Source: CAD feature listing. Evaluate the final solid. Frame: model axes, mm. Face numbers are marked on the shaded views. Give positions to 0.01 mm unless a question says otherwise; leave off trailing zeros. Order: outer loops, then holes, each group sorted by start corner. A loop starts at its lowest first (then second) coordinate and runs counter-clockwise, first axis right, second up. Notation, with made-up numbers: (55.25, -18.5) - (96.25, -18.5) arc R13 cw to (96.25, 5.5) - close; hole circle Ø9 at (27.25, -9.5). An arc over 180 degrees is marked (long way). Write each question's results on one line, items separated by ' | '. Start each with the question number.
Item 1: Section A-A on x = -10.75. Output: boundary loops of the cut face in (y, z), and give its area (3 significant figures).
Item 2: Section B-B on y = 0. Output: boundary loops of the cut face in (x, z) (3 decimals), and give its area (3 significant figures).
Item 3: Section D-D on x = 10.75. Output: boundary loops of the cut face in (y, z) (3 decimals), and give its area (3 significant figures).
Item 4: Section C-C on z = 17.5. Output: boundary loops of the cut face in (x, y).
Item 5: Line query: line 1 along Y through (x, z) = (-10.75, 12.75); line 2 along X through (y, z) = (-2, 14); line 3 along X through (y, z) = (-0.5, 6.75). Output: solid intervals per line, ascending.
Item 6: Mould query, pull axis X, two halves, no side actions, for the marked faces 1, 2, 3 and 4. Classes: released by +X, released by -X, zero draft, split by the parting line, or undercut.
```python
from build123d import *

# Parameters (mm, degrees)
SKETCH_1_W                   = 40
SKETCH_1_H                   = 20
EXTRUDE_1_DEPTH              = 20
HOLE_WIZARD_M6_1_D           = 5
HOLE_WIZARD_M6_1_CSINK_D     = 6.05
HOLE_WIZARD_M6_1_CSINK_ANGLE = 90
SKETCH_3_R                   = 3
CUT_EXTRUDE_1_DEPTH          = 31


with BuildPart() as part:
    # 草图1 → 凸台-拉伸1 (new body)
    with BuildSketch(Plane.XY):
        Rectangle(SKETCH_1_W, SKETCH_1_H)
    extrude(amount=EXTRUDE_1_DEPTH)

    # M6 螺纹孔1 (through all)
    with Locations(Plane(origin=(10.75, 0, 0), x_dir=(-1, 0, 0), z_dir=(0, 0, -1))):
        with Locations((0, 0)):
            CounterSinkHole(HOLE_WIZARD_M6_1_D / 2, HOLE_WIZARD_M6_1_CSINK_D / 2, counter_sink_angle=HOLE_WIZARD_M6_1_CSINK_ANGLE)

    # 草图3 → 切除-拉伸1 (cut, through all)
    with BuildSketch(Plane.XY.offset(20)):
        with Locations((-10.75, 0)):
            Circle(SKETCH_3_R)
    extrude(amount=-CUT_EXTRUDE_1_DEPTH, mode=Mode.SUBTRACT)


solid = part.part
```
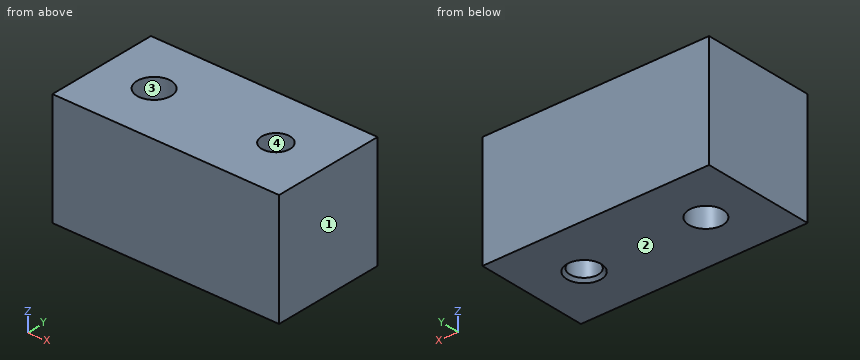
Evaluation:
1) outline: (-10, 0) - (-3, 0) - (-3, 20) - (-10, 20) - close; (3, 0) - (10, 0) - (10, 20) - (3, 20) - close | area: 280 mm^2
2) outline: (-20, 0) - (-13.75, 0) - (-13.75, 20) - (-20, 20) - close; (-7.75, 0) - (7.725, 0) - (8.25, 0.525) - (8.25, 20) - (-7.75, 20) - close; (13.25, 0.525) - (13.775, 0) - (20, 0) - (20, 20) - (13.25, 20) - close | area: 580 mm^2
3) outline: (-10, 0) - (-3.025, 0) - (-2.5, 0.525) - (-2.5, 20) - (-10, 20) - close; (2.5, 0.525) - (3.025, 0) - (10, 0) - (10, 20) - (2.5, 20) - close | area: 300 mm^2
4) outline: (-20, -10) - (20, -10) - (20, 10) - (-20, 10) - close; hole circle Ø6 at (-10.75, 0); hole circle Ø5 at (10.75, 0)
5) line 1: y = -10 to -3, 3 to 10 | line 2: x = -20 to -12.99, -8.51 to 9.25, 12.25 to 20 | line 3: x = -20 to -13.71, -7.79 to 8.3, 13.2 to 20
6) face 1: released by +X | face 2: zero draft | face 3: undercut | face 4: undercut
